Autodesk Inventor part; units mm, degrees
ref_plane "YZ Plane" through (0, 0, 0) normal (1, 0, 0) x (0, 1, 0)
ref_plane "XZ Plane" through (0, 0, 0) normal (0, 1, 0) x (-1, 0, 0)
ref_plane "XY Plane" through (0, 0, 0) normal (0, 0, 1) x (1, 0, 0)
sketch "スケッチ1" plane through (0, 0, 0) normal (0, 0, 1) x (1, 0, 0)
  circle A0 centre (0, 0) radius 23.5
  dimension "d0" = 47
extrude "押し出し1" add sketch "スケッチ1" along normal blind 5
sketch "スケッチ2" plane through (0, 0, 5) normal (0, 0, 1) x (1, 0, 0)
  circle A0 centre (0, 0) radius 15.18
  point P0 (0, 15.18)
  point P1 (-13.1463, 7.59)
  point P2 (-13.1463, -7.59)
  point P3 (0, -15.18)
  point P4 (13.1463, -7.59)
  point P5 (13.1463, 7.59)
  dimension "d3" = 30.36
  dimension "d6" = 360
hole "穴1" at (0, 15.18, 5) at (-13.1463, 7.59, 5) at (-13.1463, -7.59, 5) at (0, -15.18, 5) at (13.1463, -7.59, 5) at (13.1463, 7.59, 5) direction (0, 0, -1) diameter 4.3 end through all
sketch "スケッチ3" plane through (0, 0, 5) normal (0, 0, 1) x (1, 0, 0)
  circle A0 centre (0, 0) radius 10.1
  dimension "d15" = 20.2
extrude "押し出し2" cut sketch "スケッチ3" against normal blind 5
properties part number "servoplate_forR3" material "アルミニウム 6061"
Check sheet for the modelled part. Datum: model origin and axes. Units: mm. Round coordinates to 2 decimals unless told otherwise and drop trailing zeros. Loops run counter-clockwise (first coordinate to the right, second up) from the corner with the lowest first, then second, coordinate; pieces in that order, holes last.
1. Sectioned sample at C-C on x = -12.5. Record the boundary of the cut face in (y, z).
2. Gauge pin test, flat ends, axial feed: pin 1 Ø3.5 at (x, y) = (13.15, -7.59) entering from +Z; pin 2 Ø1.5 at (y, z) = (-13.5, 1) entering from -X; pin 3 Ø2 at (x, z) = (16, 1.5) entering from +Y. Record the tip position at first contact, or that the pin passes through.
3. Sectioned sample at B-B on y = 7.59. Record the boundary of the cut face in (x, z), and give its area (3 significant figures).
4. Mould release check, pull along Y, two halves, no side actions. Record for faces 1 (the cylindrical face through (14.45, -5.88, 2.46)), 2 (the flat face through (10, -5, 5)), 3 (the cylindrical face through (22.4, -7.1, 2.5)): released by +Y, released by -Y, zero draft, split by the parting line, or undercut.
5. Sectioned sample at D-D on y = 15.18. Record the boundary of the cut face in (x, z), and give its area (3 significant figures).
6. Scan lines: probe 1 along Y at (x, z) = (0, 3.7); probe 2 along X at (y, z) = (-7, 3.15); probe 3 along X at (y, z) = (-7.59, 2.6). Record each from-to range of solid material in increasing order.
7. Sectioned sample at A-A on x = 0. Record the boundary of the cut face in (y, z), and give its area (3 significant figures).
Recorded:
1. outline: (-19.9, 0) - (-9.64, 0) - (-9.64, 5) - (-19.9, 5) - close; (-5.54, 0) - (5.54, 0) - (5.54, 5) - (-5.54, 5) - close; (9.64, 0) - (19.9, 0) - (19.9, 5) - (9.64, 5) - close
2. pin 1: passes through
2. pin 2: stops at x = -19.74
2. pin 3: stops at y = 18.09
3. outline: (-22.24, 0) - (-15.3, 0) - (-15.3, 5) - (-22.24, 5) - close; (-11, 0) - (-6.66, 0) - (-6.66, 5) - (-11, 5) - close; (6.66, 0) - (11, 0) - (11, 5) - (6.66, 5) - close; (15.3, 0) - (22.24, 0) - (22.24, 5) - (15.3, 5) - close
3. area: 113 mm2
4. face 1: undercut
4. face 2: zero draft
4. face 3: split by the parting line
5. outline: (-17.94, 0) - (-2.15, 0) - (-2.15, 5) - (-17.94, 5) - close; (2.15, 0) - (17.94, 0) - (17.94, 5) - (2.15, 5) - close
5. area: 158 mm2
6. probe 1: y = -23.5 to -17.33, -13.03 to -10.1, 10.1 to 13.03, 17.33 to 23.5
6. probe 2: x = -22.43 to -15.21, -11.08 to -7.28, 7.28 to 11.08, 15.21 to 22.43
6. probe 3: x = -22.24 to -15.3, -11 to -6.66, 6.66 to 11, 15.3 to 22.24
7. outline: (-23.5, 0) - (-17.33, 0) - (-17.33, 5) - (-23.5, 5) - close; (-13.03, 0) - (-10.1, 0) - (-10.1, 5) - (-13.03, 5) - close; (10.1, 0) - (13.03, 0) - (13.03, 5) - (10.1, 5) - close; (17.33, 0) - (23.5, 0) - (23.5, 5) - (17.33, 5) - close
7. area: 91.0 mm2
